```python
from build123d import *

# Parameters (mm, degrees)
AUFSATZ_LINEAR_AUSTRAGEN1_DEPTH             = 15
AUFSATZ_LINEAR_AUSTRAGEN4_DEPTH             = 1.5
AUFSATZ_LINEAR_AUSTRAGEN4_DIRECTION_2_REACH = 78.164
SKIZZE6_R                                   = 1.25
SKIZZE6_W                                   = 15
SKIZZE6_H                                   = 1.5
SCHNITT_LINEAR_AUSTRAGEN1_DEPTH             = 152.28863143


with BuildPart() as part:
    # Skizze1 → Aufsatz-Linear austragen1 (new body)
    with BuildSketch(Plane.XY):
        Polygon((-74, 0), (-74, -10), (-56, -10), (-56, -5), (56, -5), (56, -10), (74, -10), (74, 0), align=None)
    extrude(amount=AUFSATZ_LINEAR_AUSTRAGEN1_DEPTH)

    # Skizze5 → Aufsatz-Linear austragen4 (add)
    with BuildSketch(Plane.XZ.offset(10)):
        Polygon((56, 0), (55, 0), (55, -1), (56, -1), (75, -1), (75, 16), (56, 16), (55, 16), (55, 15), (56, 15), (74, 15), (74, 0), align=None)
    aufsatz_linear_austragen4 = extrude(amount=AUFSATZ_LINEAR_AUSTRAGEN4_DEPTH)

    # Aufsatz-Linear austragen4 direction 2: up to this face of the body (flat: up to its plane)
    aufsatz_linear_austragen4_direction_2_end = Plane(part.part.faces().sort_by_distance((0, 0, 7.5))[0])
    # Skizze5 → Aufsatz-Linear austragen4 direction 2 (add, up to the picked face)
    with BuildSketch(Plane.XZ.offset(10), mode=Mode.PRIVATE) as aufsatz_linear_austragen4_direction_2_sk1:
        Polygon((56, 0), (55, 0), (55, -1), (56, -1), (75, -1), (75, 16), (56, 16), (55, 16), (55, 15), (56, 15), (74, 15), (74, 0), align=None)
    aufsatz_linear_austragen4_direction_2_tool1 = split(extrude(aufsatz_linear_austragen4_direction_2_sk1.sketch, amount=-AUFSATZ_LINEAR_AUSTRAGEN4_DIRECTION_2_REACH, mode=Mode.PRIVATE), bisect_by=aufsatz_linear_austragen4_direction_2_end, keep=Keep.BOTH, mode=Mode.PRIVATE)
    aufsatz_linear_austragen4_direction_2 = aufsatz_linear_austragen4_direction_2_tool1.solids().sort_by(Axis((55.5, -10, -0.262488), (0, 1, 0)))[0]
    add(aufsatz_linear_austragen4_direction_2)

    # Spiegeln1: Aufsatz-Linear austragen4, Aufsatz-Linear austragen4 direction 2 across plane
    add(aufsatz_linear_austragen4.mirror(Plane(origin=(0, 0, 0), x_dir=(0, 0, 1), z_dir=(1, 0, 0))))
    add(aufsatz_linear_austragen4_direction_2.mirror(Plane(origin=(0, 0, 0), x_dir=(0, 0, 1), z_dir=(1, 0, 0))))

    # Skizze6 → Schnitt-Linear austragen1 (cut, through all)
    with BuildSketch(Plane.ZY.offset(75)):
        with Locations(Location((10, -2, 0), (0, 0, 270))):
            Circle(SKIZZE6_R)
        with Locations(Location((5, -2, 0), (0, 0, 90))):
            Circle(SKIZZE6_R)
        with Locations((7.5, -10.75)):
            Rectangle(SKIZZE6_W, SKIZZE6_H)
    extrude(amount=-SCHNITT_LINEAR_AUSTRAGEN1_DEPTH, mode=Mode.SUBTRACT)


solid = part.part
```
Input: part model. Units: mm. Frame: model coordinates. A direction names the side the tool comes from. Round coordinates to 2 decimals unless told otherwise and drop trailing zeros. Loops run counter-clockwise (first coordinate to the right, second up) from the corner with the lowest first, then second, coordinate; pieces in that order, holes last. Notation, with made-up numbers: M 68,70 L 74,70 A19 ccw 74,106 Z; hole C 28.25,49.5 d8. An arc over 180 degrees is marked long. Answer in a Markdown table with one row per item. Add a question column.
1. Set-up query: faces 4 (the face through (-1, -2, 15)), 5 (the face through (-66, -10, 7)), 6 (the face through (-1, -2, 0)), 7 (the face through (63.5, -10.2, 15)). Return all of +Z, -Z, +X, -X, +Y, -Y with unobstructed straight access to the full face (end or side cutting, diameter ignored); none if empty.
2. Contact query for flat-ended pins moving along their axis: pin 1 (2.5 mm diameter, centred on x = -7, y = -3, fed in from -Z); pin 2 (5 mm diameter, centred on x = -22.5, y = -3, fed in from +Z); pin 3 (5 mm diameter, centred on x = 3.5, y = -8.5, fed in from +Z); pin 4 (7.5 mm diameter, centred on x = 65.5, z = 5.5, fed in from -Y). Output: stop coordinate, or through.
3. Section C-C (x = -5). Output: boundary loops of the cut face in (y, z), and give its area (3 significant figures).
4. Mould query, pull axis Y, two halves, no side actions, for faces 1 (the face through (-1.05, -1.423, 6.109)), 2 (the face through (-75, -6, 7)), 3 (the face through (-1, 0, 8)). Classes: released by +Y, released by -Y, zero draft, split by the parting line, or undercut.
5. Section B-B (z = 5). Output: boundary loops of the cut face in (x, y), and give its area (3 significant figures).
6. Section A-A (y = -2). Output: boundary loops of the cut face in (x, z), and give its area (3 significant figures).
7. Ray query, probe 1 along Z at (x, y) = (-39, -2); probe 2 along Y at (x, z) = (37, 5); probe 3 along X at (y, z) = (-7.5, 7.5). Return the intervals inside material, ascending.
Values follow:
| question | item | result |
|---|---|---|
| 1 | face 4 | +Z, +Y, -Y |
| 1 | face 5 | +X, -X, -Y |
| 1 | face 6 | -Z, +Y, -Y |
| 1 | face 7 | -Y |
| 2 | pin 1 | z = 0 |
| 2 | pin 2 | z = 15 |
| 2 | pin 3 | through |
| 2 | pin 4 | y = -10 |
| 3 | outline | M -5,0 L 0,0 L 0,15 L -5,15 Z; hole C -2,5 d2.5; hole C -2,10 d2.5 |
| 3 | area | 65.2 mm^2 |
| 4 | face 1 | undercut |
| 4 | face 2 | zero draft |
| 4 | face 3 | released by +Y |
| 5 | outline | M -75,-10 L -56,-10 L -56,-5 L 56,-5 L 56,-10 L 75,-10 L 75,-3.25 L -75,-3.25 Z; M -75,-0.75 L 75,-0.75 L 75,0 L -75,0 Z |
| 5 | area | 565 mm^2 |
| 6 | outline | M -75,-1 L -55,-1 L -55,0 L 55,0 L 55,-1 L 75,-1 L 75,3.75 L -75,3.75 Z; M -75,6.25 L 75,6.25 L 75,8.75 L -75,8.75 Z; M -75,11.25 L 75,11.25 L 75,16 L 55,16 L 55,15 L -55,15 L -55,16 L -75,16 Z |
| 6 | area | 1,580 mm^2 |
| 7 | probe 1 | 0 to 3.75, 6.25 to 8.75, 11.25 to 15 |
| 7 | probe 2 | -5 to -3.25, -0.75 to 0 |
| 7 | probe 3 | -75 to -56, 56 to 75 |
